Geometry check sheet. Reference: drawing and pictorial views, mm from the part's lowest x, y, z. A direction names the side the tool comes from. Give positions to 0.01 mm unless a question says otherwise; leave off trailing zeros. Order: outer loops, then holes, each group sorted by start corner. A loop starts at its lowest first (then second) coordinate and runs counter-clockwise, first axis right, second up. Notation, with made-up numbers: (14, 75.25) -> (28, 75.25) arc R24 cw to (28, 86.25) -> close; hole circle Ø10 at (87.5, -32.5). An arc over 180 degrees is marked (long way). Write each question's results on one line, items separated by ' | '. Start each with the question number.
1. Cross-section at D-D, the plane x = 25. Enter the section's corners in (y, z) (1 decimal).
2. Material ranges on L1, parallel to X at y = 28, z = 9.5 (1 decimal); L2, parallel to Z at x = 17.5, y = 28; L3, parallel to Y at x = 24, z = 11 (1 decimal), recorded low to high. Write a range as from..to.
3. Set-up check for the marked faces 1 and 2: record each of +Z, -Z, +X, -X, +Y, -Y from which the full face is reachable in a straight line by a thin tool's end or side.
4. Cross-section at B-B, the plane y = 18. Enter the section's corners in (x, z).
5. Depth check by flat-ended pin: pin 1 Ø3 at (x, z) = (28.5, 6.5) entering from -Y; pin 2 Ø2 at (x, y) = (24, 13.5) entering from +Z; pin 3 Ø5 at (x, z) = (7, 6) entering from -Y (1 decimal). Enter the tip coordinate at first touch or a pass-through.
6. Cross-section at C-C, the plane x = 17.5. Enter the section's corners in (y, z) (1 decimal), then the cut area to 3 significant figures.
7. Cross-section at A-A, the plane z = 1. Enter the section's corners in (x, y) (1 decimal), then the cut area to 3 significant figures.
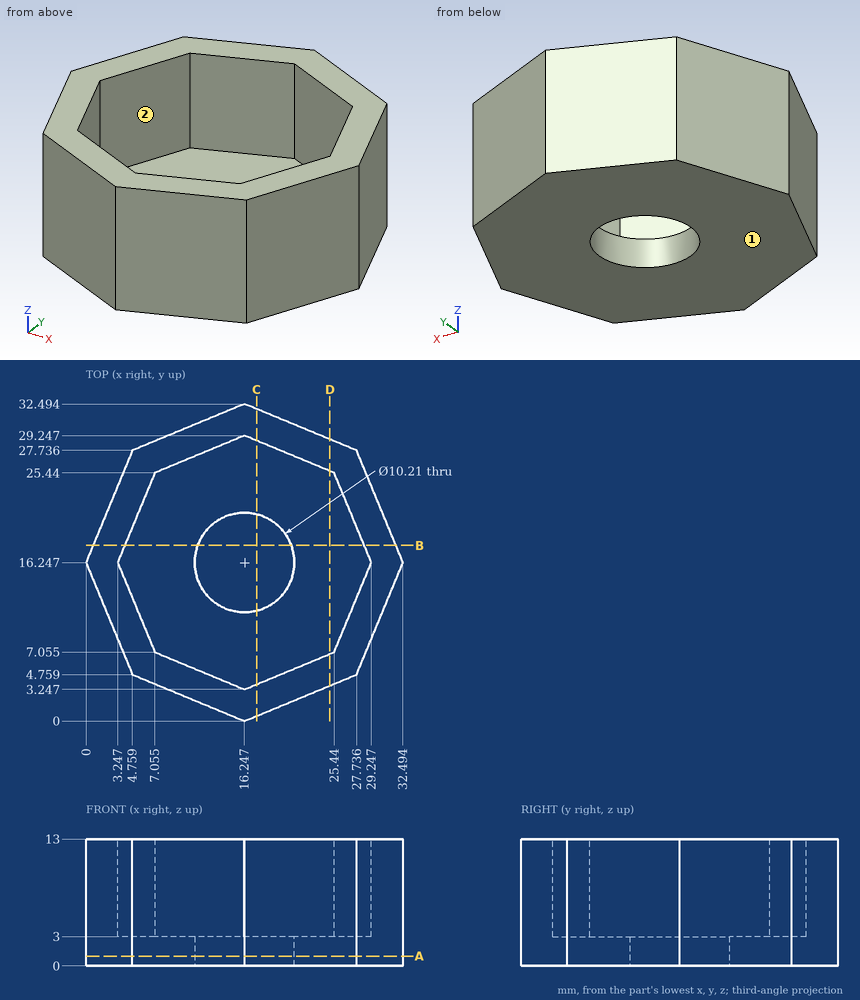
Results below:
1) outline: (3.6, 0) -> (28.9, 0) -> (28.9, 13) -> (25.6, 13) -> (25.6, 3) -> (6.9, 3) -> (6.9, 13) -> (3.6, 13) -> close
2) L1: x = 5.4..13.2, 19.3..27.1 | L2: z = 0..3 | L3: y = 3.2..6.5, 26..29.3
3) face 1: -Z, +X, -X, +Y, -Y | face 2: +Z
4) outline: (0.73, 0) -> (11.45, 0) -> (11.45, 3) -> (3.97, 3) -> (3.97, 13) -> (0.73, 13) -> close; (21.04, 0) -> (31.77, 0) -> (31.77, 13) -> (28.52, 13) -> (28.52, 3) -> (21.04, 3) -> close
5) pin 1: stops at y = 4.45 | pin 2: stops at z = 3 | pin 3: stops at y = 2.8
6) outline: (0.5, 0) -> (11.3, 0) -> (11.3, 3) -> (3.8, 3) -> (3.8, 13) -> (0.5, 13) -> close; (21.2, 0) -> (32, 0) -> (32, 13) -> (28.7, 13) -> (28.7, 3) -> (21.2, 3) -> close | area: 130 mm²
7) outline: (0, 16.2) -> (4.8, 4.8) -> (16.2, 0) -> (27.7, 4.8) -> (32.5, 16.2) -> (27.7, 27.7) -> (16.2, 32.5) -> (4.8, 27.7) -> close; hole circle Ø10.2 at (16.2, 16.2) | area: 665 mm²
